```python
from build123d import *

# Parameters (mm, degrees)
BOSS_SWITCH_BODY_DEPTH            = 3
SKETCH1_W                         = 2.994375291
SKETCH1_H                         = 2.409101515
SKETCH1_W_2                       = 3.994375291
SKETCH1_H_2                       = 3.957767538
BOSS_FLANGE_WIDTH_DEPTH           = 5
BOSS_FLANGE_HEIGHT_REACH          = 36.354
SKETCH2_W                         = 4
SKETCH2_H                         = 3.957767538
SKETCH2_W_2                       = 8
SKETCH2_H_2                       = 1.451333978
SKETCH17_W                        = 15.1675
SKETCH17_H                        = 4
BOSS_FLANGE_SUPPORT_DEPTH         = 13.053634428
CUT_WALL_GAP_DEPTH                = 1
TAP_DRILL_FOR_M2X0_4_TAP1_D       = 1.6
M2_CLEARANCE_HOLE2_D              = 2.4
M2_CLEARANCE_HOLE2_DEPTH          = 13.462735941
CHAMFER_FLANGE_SUPPORT_3_SIZE     = 1
FILLET1_R                         = 1
FILLET2_R                         = 0.5
SKETCH28_W                        = 5.9675
SKETCH28_H                        = 12.095866891
CUT_PRINT_SUPPORT_CLEARANCE_DEPTH = 33.624103931


with BuildPart() as part:
    # Sketch-SwitchBossUp → Boss-Switch Body (new body)
    with BuildSketch(Plane.XY):
        with BuildLine():
            Line((-5.697895702, 26.949658376), (-5.524247524, 25.964850623))
            ThreePointArc((-5.524247524, 25.964850623), (-6.169751391, 25.553619307), (-6.3354071, 24.806394693))
            Line((-6.3354071, 24.806394693), (-4.07798079, 12.003893904))
            ThreePointArc((-4.07798079, 12.003893904), (-3.666749473, 11.358390037), (-2.919524859, 11.192734328))
            Line((-2.919524859, 11.192734328), (-2.775521101, 10.376048434))
            Line((-2.775521101, 10.376048434), (-1.884274871, 10.03057987))
            Line((-1.884274871, 10.03057987), (-1.254903211, 9.786620214))
            Line((-1.254903211, 9.786620214), (-1.735258621, 8.547390389))
            ThreePointArc((-1.735258621, 8.547390389), (-1.752158006, 8.457034961), (-1.735258621, 8.366679532))
            Line((-1.735258621, 8.366679532), (-1.254903211, 7.127449707))
            Line((-1.254903211, 7.127449707), (-1.884274871, 6.883490051))
            Line((-1.884274871, 6.883490051), (-0.547014535, 3.433600952))
            Line((-0.547014535, 3.433600952), (0.082357125, 3.677560608))
            Line((0.082357125, 3.677560608), (0.805200549, 1.81275569))
            Line((0.805200549, 1.81275569), (-0.12720191, 1.451333978))
            Line((-0.12720191, 1.451333978), (-0.12720191, 0))
            Line((-0.12720191, 0), (2.867173381, 0))
            Line((2.867173381, 0), (2.867173381, 2.409101515))
            Line((2.867173381, 2.409101515), (2.343664607, 2.409101515))
            Line((2.343664607, 2.409101515), (1.411262148, 2.047679803))
            Line((1.411262148, 2.047679803), (0.688418723, 3.912484721))
            Line((0.688418723, 3.912484721), (1.317790383, 4.156444377))
            Line((1.317790383, 4.156444377), (1.099194858, 4.720381179))
            Line((1.099194858, 4.720381179), (3.161331824, 5.519715271))
            Line((3.161331824, 5.519715271), (3.161331824, 6.855167315))
            Line((3.161331824, 6.855167315), (2.261147576, 7.841686204))
            Line((2.261147576, 7.841686204), (0.199125572, 7.042396674))
            Line((0.199125572, 7.042396674), (-0.019469953, 7.606333476))
            Line((-0.019469953, 7.606333476), (-0.648841612, 7.36237382))
            Line((-0.648841612, 7.36237382), (-1.038134762, 8.366679532))
            ThreePointArc((-1.038134762, 8.366679532), (-1.055034148, 8.457034961), (-1.038134762, 8.547390389))
            Line((-1.038134762, 8.547390389), (-0.648841612, 9.551696101))
            Line((-0.648841612, 9.551696101), (-0.019469953, 9.307736445))
            Line((-0.019469953, 9.307736445), (1.317790383, 12.757625544))
            Line((1.317790383, 12.757625544), (0.688418723, 13.0015852))
            Line((0.688418723, 13.0015852), (1.411262148, 14.866390118))
            Line((1.411262148, 14.866390118), (2.343664607, 14.504968406))
            Line((2.343664607, 14.504968406), (2.867173381, 14.504968406))
            Line((2.867173381, 14.504968406), (2.867173381, 18.462735944))
            Line((2.867173381, 18.462735944), (-0.111637615, 18.462735944))
            Line((-0.111637615, 18.462735944), (-1.12720191, 18.462735944))
            Line((-1.12720191, 18.462735944), (-1.12720191, 15.462735944))
            Line((-1.12720191, 15.462735944), (-0.12720191, 15.462735944))
            Line((-0.12720191, 15.462735944), (0.805200549, 15.101314231))
            Line((0.805200549, 15.101314231), (0.082357125, 13.236509313))
            Line((0.082357125, 13.236509313), (-0.547014535, 13.480468969))
            Line((-0.547014535, 13.480468969), (-1.059112089, 12.159350171))
            Line((-1.059112089, 12.159350171), (-2.346896051, 19.462735944))
            Line((-2.346896051, 19.462735944), (3.767173381, 19.462735944))
            Line((3.767173381, 19.462735944), (3.767173381, 25.857619356))
            Line((3.767173381, 25.857619356), (1.767173381, 25.857619356))
            Line((1.767173381, 25.857619356), (1.767173381, 21.462735944))
            Line((1.767173381, 21.462735944), (-2.699550012, 21.462735944))
            Line((-2.699550012, 21.462735944), (-3.728280196, 27.296954732))
            ThreePointArc((-3.728280196, 27.296954732), (-2.874356585, 27.992742953), (-2.319025652, 28.944012807))
            ThreePointArc((-2.319025652, 28.944012807), (-2.76728001, 29.905297381), (-3.728564583, 29.457043022))
            ThreePointArc((-3.728564583, 29.457043022), (-4.944660137, 28.436617692), (-6.436422172, 28.97957467))
            ThreePointArc((-6.436422172, 28.97957467), (-7.493046212, 29.072017295), (-7.585488837, 28.015393255))
            ThreePointArc((-7.585488837, 28.015393255), (-6.738295005, 27.311426358), (-5.697895702, 26.949658376))
        make_face()
    extrude(amount=BOSS_SWITCH_BODY_DEPTH)

    # Sketch1 → Boss-Flange Width (add)
    with BuildSketch(Plane(origin=(0, 0, 0), x_dir=(-1, 0, 0), z_dir=(0, 0, -1))):
        with Locations((-1.369985736, 1.204550758)):
            Rectangle(SKETCH1_W, SKETCH1_H)
        with Locations((-0.869985736, 16.483852175)):
            Rectangle(SKETCH1_W_2, SKETCH1_H_2)
    extrude(amount=BOSS_FLANGE_WIDTH_DEPTH)

    # Boss-Flange Height: up to this face of the body (flat: up to its plane)
    boss_flange_height_end = Plane(part.part.faces().sort_by_distance((-0.12720191, 1.077409098, -1.438016547))[0])
    # Sketch2 → Boss-Flange Height (add, up to the picked face)
    with BuildSketch(Plane(origin=(-12.300326619, 0, 0), x_dir=(0, 0, -1), z_dir=(1, 0, 0)), mode=Mode.PRIVATE) as boss_flange_height_sk1:
        with Locations((3, 16.483852175)):
            Rectangle(SKETCH2_W, SKETCH2_H)
    boss_flange_height_tool1 = split(extrude(boss_flange_height_sk1.sketch, amount=BOSS_FLANGE_HEIGHT_REACH, mode=Mode.PRIVATE), bisect_by=boss_flange_height_end, keep=Keep.BOTH, mode=Mode.PRIVATE)
    # Sketch2 → Boss-Flange Height (add, up to the picked face)
    with BuildSketch(Plane(origin=(-12.300326619, 0, 0), x_dir=(0, 0, -1), z_dir=(1, 0, 0)), mode=Mode.PRIVATE) as boss_flange_height_sk2:
        with Locations((1, 0.725666989)):
            Rectangle(SKETCH2_W_2, SKETCH2_H_2)
    boss_flange_height_tool2 = split(extrude(boss_flange_height_sk2.sketch, amount=BOSS_FLANGE_HEIGHT_REACH, mode=Mode.PRIVATE), bisect_by=boss_flange_height_end, keep=Keep.BOTH, mode=Mode.PRIVATE)
    add(boss_flange_height_tool1.solids().sort_by(Axis((-12.300327, 16.483852, -3), (1, 0, 0)))[0])
    add(boss_flange_height_tool2.solids().sort_by(Axis((-12.300327, 0.725667, -1), (1, 0, 0)))[0])

    # Sketch17 → Boss-Flange Support (add)
    with BuildSketch(Plane.XZ.offset(-1.451333978)):
        with Locations((-4.716576619, -3)):
            Rectangle(SKETCH17_W, SKETCH17_H)
    extrude(amount=-BOSS_FLANGE_SUPPORT_DEPTH)

    # Sketch27 → Cut-Wall Gap (cut)
    with BuildSketch(Plane.XY):
        Polygon((-0.12720191, 15.462735944), (2.343664607, 14.504968406), (-1.12720191, 14.504968406), (-1.12720191, 15.462735944), align=None)
        Polygon((2.343664607, 2.409101515), (-0.12720191, 2.409101515), (-0.12720191, 1.451333978), align=None)
    extrude(amount=-CUT_WALL_GAP_DEPTH, mode=Mode.SUBTRACT)

    # Tap Drill for M2x0.4 Tap1 (through all)
    with Locations(Plane(origin=(0, 0, 0), x_dir=(-1, 0, 0), z_dir=(0, -1, 0))):
        with Locations((9.300326619, 3), (5.300326619, 3)):
            Hole(TAP_DRILL_FOR_M2X0_4_TAP1_D / 2)

    # M2 Clearance Hole2
    with Locations(Plane.XZ):
        with Locations((-9.300326619, -3), (-5.300326619, -3)):
            Hole(M2_CLEARANCE_HOLE2_D / 2, depth=M2_CLEARANCE_HOLE2_DEPTH)

    # Chamfer-Flange Support 3
    chamfer_flange_support_3_edges = [part.edges().sort_by_distance(p)[0] for p in [
        (-6.213764264, 1.451333978, -1),
    ]]
    chamfer(chamfer_flange_support_3_edges, length=CHAMFER_FLANGE_SUPPORT_3_SIZE)

    # Fillet1
    fillet1_edges = [part.edges().sort_by_distance(p)[0] for p in [
        (-2.775521101, 10.376048434, 1.5),
    ]]
    fillet(fillet1_edges, radius=FILLET1_R)

    # Fillet2
    fillet2_edges = [part.edges().sort_by_distance(p)[0] for p in [
        (-1.884274871, 6.883490051, 1.5),
    ]]
    fillet(fillet2_edges, radius=FILLET2_R)

    # Sketch28 → Cut-Print Support Clearance (cut, through all)
    with BuildSketch(Plane.XY.offset(-1)):
        with Locations((-0.116576619, 8.457034961)):
            Rectangle(SKETCH28_W, SKETCH28_H)
    extrude(amount=-CUT_PRINT_SUPPORT_CLEARANCE_DEPTH, mode=Mode.SUBTRACT)


solid = part.part
```
CAD build for the part. Positions are in the model's coordinates, mm. A direction names the side the tool comes from. Round coordinates to 2 decimals unless told otherwise and drop trailing zeros. Loops run counter-clockwise (first coordinate to the right, second up) from the corner with the lowest first, then second, coordinate; pieces in that order, holes last. Notation, with made-up numbers: M 77.5,88.25 L 123.5,88.25 A15 cw 123.5,117.25 Z; hole C 33,19 d8. An arc over 180 degrees is marked long. Return JSON: item names as keys, results as strings. Group by question number.
(1) Saw through at A-A, the plane z = -3. List the corners of the cut face in (x, y).
(2) Wall check: probe 1 along X at (y, z) = (16.1, -3); probe 2 along Y at (x, z) = (-3, -1.75); probe 3 along Y at (x, z) = (-2.5, 2.25). Give the ranges that are in metal, low to high. Write a range as [from, to].
(3) Drop flat-ended pins along their axis: P1, Ø3, axis at y = 16.5, z = -1, coming from the +X side; P2, Ø0.9, axis at x = -1, z = 1.5, coming from the +Y side; P3, Ø0.7, axis at x = -9.5, z = -2.5, coming from the -Y side; P4, Ø1.3, axis at x = -5.3, z = -3, coming from the +Y side. Give the stop position or say it passes through.
(4) Mould opens along X. For faces 5 (the flat face through (-1.49, 9.18, 1.48)), 6 (the flat face through (-0.6, 15.463, 1)), 7 (the flat face through (2.116, 5.114, 1.479)), 8 (the cylindrical face through (-2.75, 29.9, 1.48)) say: +X half, -X half, draft (parallel to the pull), parting line (faces both ways), or undercut.
(5) Tool access for faces 1 (the flat face through (-5, 13.463, -4)), 2 (the flat face through (1.245, 7.448, 1.479)), 3 (the flat face through (-1.5, 7.76, 1.48)), 4 (the flat face through (1, 19.463, 1)): list every direction of +Z, -Z, +X, -X, +Y, -Y with a clear straight run to the whole face (end or side of a thin tool).
(6) Saw through at D-D, the plane z = -4.5. List the corners of the cut face in (x, y).
(7) Saw through at B-B, the plane y = 17.5. List the corners of the cut face in (x, z).
(8) Saw through at C-C, the plane y = 24.5. List the corners of the cut face in (x, z), and give its area (3 significant figures).
Answer list:
{
 "1": {"outline": "M -12.3,0 L -10.5,0 L -10.5,13.46 L -10.1,13.46 L -10.1,18.46 L -12.3,18.46 Z; M -8.5,13.46 L -8.1,13.46 L -8.1,0 L -6.5,0 L -6.5,13.46 L -6.1,13.46 L -6.1,18.46 L -8.5,18.46 Z; M -4.5,13.46 L -4.1,13.46 L -4.1,0 L 2.87,0 L 2.87,2.41 L -3.1,2.41 L -3.1,14.5 L 2.87,14.5 L 2.87,18.46 L -4.5,18.46 Z"},
 "2": {"probe 1": "[-12.3, -10.1], [-8.5, -6.1], [-4.5, 2.87]", "probe 2": "[0, 2.41], [14.5, 18.46]", "probe 3": "[0, 1.45], [10.31, 21.46], [28.54, 29.74]"},
 "3": {"P1": "x = 2.87", "P2": "y = 21.46", "P3": "y = 13.46", "P4": "through"},
 "4": {"face 5": "-X half", "face 6": "undercut", "face 7": "+X half", "face 8": "parting line"},
 "5": {"face 1": "-Y", "face 2": "+Z, -Z", "face 3": "+Z, -Z, -X", "face 4": "+Z, -Z, +X"},
 "6": {"outline": "M -12.3,0 L 2.87,0 L 2.87,2.41 L -3.1,2.41 L -3.1,14.5 L 2.87,14.5 L 2.87,18.46 L -12.3,18.46 Z"},
 "7": {"outline": "M -12.3,-5 L 2.87,-5 L 2.87,3 L -1.13,3 L -1.13,-1 L -12.3,-1 Z; M -5.05,0 L -2,0 L -2,3 L -5.05,3 Z; hole C -9.3,-3 d1.6; hole C -5.3,-3 d1.6"},
 "8": {"outline": "M -6.28,0 L -3.24,0 L -3.24,3 L -6.28,3 Z; M 1.77,0 L 3.77,0 L 3.77,3 L 1.77,3 Z", "area": "15.1 mm2"}
}
